```python
from build123d import *

# Parameters (mm, degrees)
F1_DEPTH = 10.16


with BuildPart() as f1:
    # F0 (on Front) → F1 (new body)
    with BuildSketch(Plane.XZ):
        with BuildLine():
            Line((3.175, -12.531403), (3.175, 17.285798))
            Line((3.175, 17.285798), (-3.175, 17.285798))
            ThreePointArc((-3.175, 17.285798), (-7.266525, 14.65801), (-12.065, 13.870302))
            Line((-12.065, 13.870302), (-12.065, 10.425861))
            Line((-12.065, 10.425861), (-3.175, 10.425861))
            Line((-3.175, 10.425861), (-3.175, -12.533976))
            ThreePointArc((-3.175, -12.533976), (-4.601328, -15.977436), (-8.044787, -17.403763))
            Line((-8.044787, -17.403763), (-12.323086, -17.403763))
            Line((-12.323086, -17.403763), (-12.323086, -19.825798))
            Line((-12.323086, -19.825798), (0, -19.825798))
            Line((0, -19.825798), (12.323086, -19.825798))
            Line((12.323086, -19.825798), (12.323086, -17.285798))
            Line((12.323086, -17.285798), (7.929395, -17.285798))
            ThreePointArc((7.929395, -17.285798), (4.56753, -15.893268), (3.175, -12.531403))
        make_face()
    extrude(amount=F1_DEPTH)


solid = f1.part
```
Build history of the part. All positions in model axes, mm. A direction names the side the tool comes from. Round coordinates to 2 decimals unless told otherwise and drop trailing zeros. Loops run counter-clockwise (first coordinate to the right, second up) from the corner with the lowest first, then second, coordinate; pieces in that order, holes last.
Item 1: Pin check, flat tips, straight feed: P1, Ø8, axis at x = 4, z = -4.5, coming from the +Y side; P2, Ø1.7, axis at y = -5, z = 11.5, coming from the -X side (3 decimals); P3, Ø3.5, axis at x = -10.5, y = -2.5, coming from the +Z side; P4, Ø5, axis at x = 10.5, y = -6, coming from the +Z side. Stop position of each tip, or through.
Item 2: Two-plate mould, pull along Z, no slides. Class faces 1 (the face through (-4.564, -5.009, -15.939)), 2 (the face through (12.323, -5, -19)), 3 (the face through (4.605, -5.009, -15.93)): released by +Z, released by -Z, zero draft, split by the parting line, or undercut.
Item 3: Saw through at B-B (y = -3). List the corners of the cut face in (x, z) (3 decimals), then the cut area to 3 significant figures.
Item 4: Which spindle directions (+Z, -Z, +X, -X, +Y, -Y) get a long thin tool onto all of the face, cutting with end or side? Do faces 4 (the face through (3.175, -5, 2)), 5 (the face through (-12.065, -5, 12)), 6 (the face through (-10, -5, -17.404)). Say none if no direction does.
Item 5: Drill centre lines: line 1 along X through (y, z) = (-4.25, 6) (3 decimals); line 2 along Z through (x, y) = (11.25, -2.5); line 3 along Z through (x, y) = (-5.25, -6.5). Where is each one in solid material? Low to high.
Item 6: Saw through at A-A (x = -6.5). List the corners of the cut face in (y, z), then the cut area to 3 significant figures.
Item 7: Saw through at C-C (z = 7). List the corners of the cut face in (x, y) (3 decimals).
Item 8: Saw through at D-D (x = 10). List the corners of the cut face in (y, z).
Worked answers:
1. P1: stops at y = 0
1. P2: stops at x = -12.065
1. P3: stops at z = 14.2
1. P4: stops at z = -17.29
2. face 1: undercut
2. face 2: zero draft
2. face 3: released by +Z
3. outline: (-12.323, -19.826) - (12.323, -19.826) - (12.323, -17.286) - (7.929, -17.286) arc R4.754 cw to (3.175, -12.531) - (3.175, 17.286) - (-3.175, 17.286) arc R11.996 cw to (-12.065, 13.87) - (-12.065, 10.426) - (-3.175, 10.426) - (-3.175, -12.534) arc R4.87 cw to (-8.045, -17.404) - (-12.323, -17.404) - close
3. area: 330 mm2
4. face 4: +Z, +X, +Y, -Y
4. face 5: +Z, -X, +Y, -Y
4. face 6: -X, +Y, -Y
5. line 1: x = -3.175 to 3.175
5. line 2: z = -19.83 to -17.29
5. line 3: z = -19.83 to -16.52, 10.43 to 15.66
6. outline: (-10.16, -19.83) - (0, -19.83) - (0, -17.15) - (-10.16, -17.15) - close; (-10.16, 10.43) - (0, 10.43) - (0, 14.98) - (-10.16, 14.98) - close
6. area: 73.5 mm2
7. outline: (-3.175, -10.16) - (3.175, -10.16) - (3.175, 0) - (-3.175, 0) - close
8. outline: (-10.16, -19.83) - (0, -19.83) - (0, -17.29) - (-10.16, -17.29) - close
